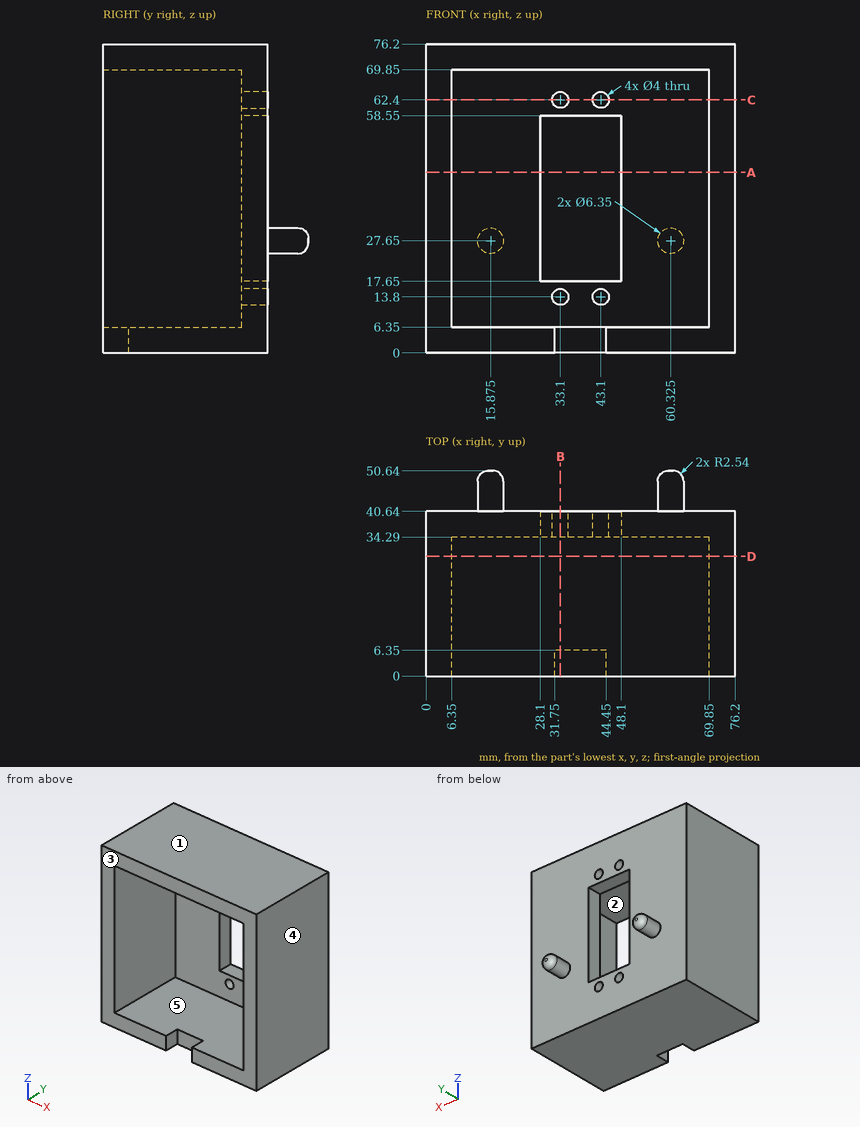
For this review, use the dimensioned drawing (mm, ordinates from the lowest corner) and the shaded views. A direction names the side the tool comes from. Round coordinates to 2 decimals unless told otherwise and drop trailing zeros. Write each loop counter-clockwise with the first axis right and the second up, starting at its lowest first coordinate (ties: lowest second). Pieces come first, ordered by that corner, then holes. Notation, with made-up numbers: (84.5, 83) -> (113.5, 83) arc R28 cw to (113.5, 114) -> close; hole circle Ø4 at (-16.5, -1.5). An arc over 180 degrees is marked (long way). Use one line per item in the form item = value.
Q1. The part is to be moulded in two halves that separate along Z. For the marked faces 1, 2 and 3, say which applies: released by +Z, released by -Z, zero draft, split by the parting line, or undercut.
Resolved:
face_1 = released by +Z
face_2 = undercut
face_3 = zero draft
Q2. Consider section A-A (z = 44.5). State the section outline as (x, y) points.
Resolved:
outline = (0, 0) -> (6.35, 0) -> (6.35, 34.29) -> (28.1, 34.29) -> (28.1, 40.64) -> (0, 40.64) -> close; (48.1, 34.29) -> (69.85, 34.29) -> (69.85, 0) -> (76.2, 0) -> (76.2, 40.64) -> (48.1, 40.64) -> close
Q3. To check wall thickness, follow probe 1 along Z at (x, y) = (43, 38); probe 2 along X at (y, z) = (37.75, 62.4); probe 3 along Z at (x, y) = (12, 33.5). State the ranges of each line that lie inside material, in increasing order. Write a range as from..to.
Resolved:
probe_1 = 0..11.8, 15.8..17.65, 58.55..60.4, 64.4..76.2
probe_2 = 0..31.1, 35.1..41.1, 45.1..76.2
probe_3 = 0..6.35, 69.85..76.2
Q4. Machinability: for the marked faces 4 and 5, which of the approach directions +Z, -Z, +X, -X, +Y, -Y give a long, thin tool a straight path to every point of the face, cutting with its end or side? Answer none if there is none.
Resolved:
face_4 = +Z, -Z, +X, +Y, -Y
face_5 = -Y
Q5. Clearance check with flat-ended pins moving along their axes: pin 1 Ø1 at (x, z) = (56.5, 15.5) entering from +Y; pin 2 Ø3 at (x, z) = (38, 4.5) entering from -Y; pin 3 Ø3.5 at (x, z) = (43.1, 62.4) entering from -Y; pin 4 Ø5 at (x, z) = (33.1, 62.4) entering from -Y. State where each tip first meets the part, or that it passes through.
Resolved:
pin_1 = 40.64
pin_2 = 6.35
pin_3 = through
pin_4 = 34.29
Q6. Consider section C-C (z = 62.4). State the section outline as (x, y) points.
Resolved:
outline = (0, 0) -> (6.35, 0) -> (6.35, 34.29) -> (31.1, 34.29) -> (31.1, 40.64) -> (0, 40.64) -> close; (35.1, 34.29) -> (41.1, 34.29) -> (41.1, 40.64) -> (35.1, 40.64) -> close; (45.1, 34.29) -> (69.85, 34.29) -> (69.85, 0) -> (76.2, 0) -> (76.2, 40.64) -> (45.1, 40.64) -> close
Q7. Consider section D-D (y = 29.5). State the section outline as (x, z) points.
Resolved:
outline = (0, 0) -> (76.2, 0) -> (76.2, 76.2) -> (0, 76.2) -> close; hole (6.35, 6.35) -> (69.85, 6.35) -> (69.85, 69.85) -> (6.35, 69.85) -> close
Q8. Consider section B-B (x = 33.1). State the section outline as (y, z) points.
Resolved:
outline = (0, 69.85) -> (34.29, 69.85) -> (34.29, 64.4) -> (40.64, 64.4) -> (40.64, 76.2) -> (0, 76.2) -> close; (6.35, 0) -> (40.64, 0) -> (40.64, 11.8) -> (34.29, 11.8) -> (34.29, 6.35) -> (6.35, 6.35) -> close; (34.29, 15.8) -> (40.64, 15.8) -> (40.64, 17.65) -> (34.29, 17.65) -> close; (34.29, 58.55) -> (40.64, 58.55) -> (40.64, 60.4) -> (34.29, 60.4) -> close
